Can you work these out from the drawing? Everything is in mm from the part's minimum corner. A direction names the side the tool comes from. Round coordinates to 2 decimals unless told otherwise and drop trailing zeros. Loops run counter-clockwise (first coordinate to the right, second up) from the corner with the lowest first, then second, coordinate; pieces in that order, holes last. Notation, with made-up numbers: M -7,-3.5 L 18,-3.5 A33 cw 18,25.5 Z; hole C 86.25,86.25 d8. An arc over 180 degrees is marked long. Use a Markdown table: item, result.
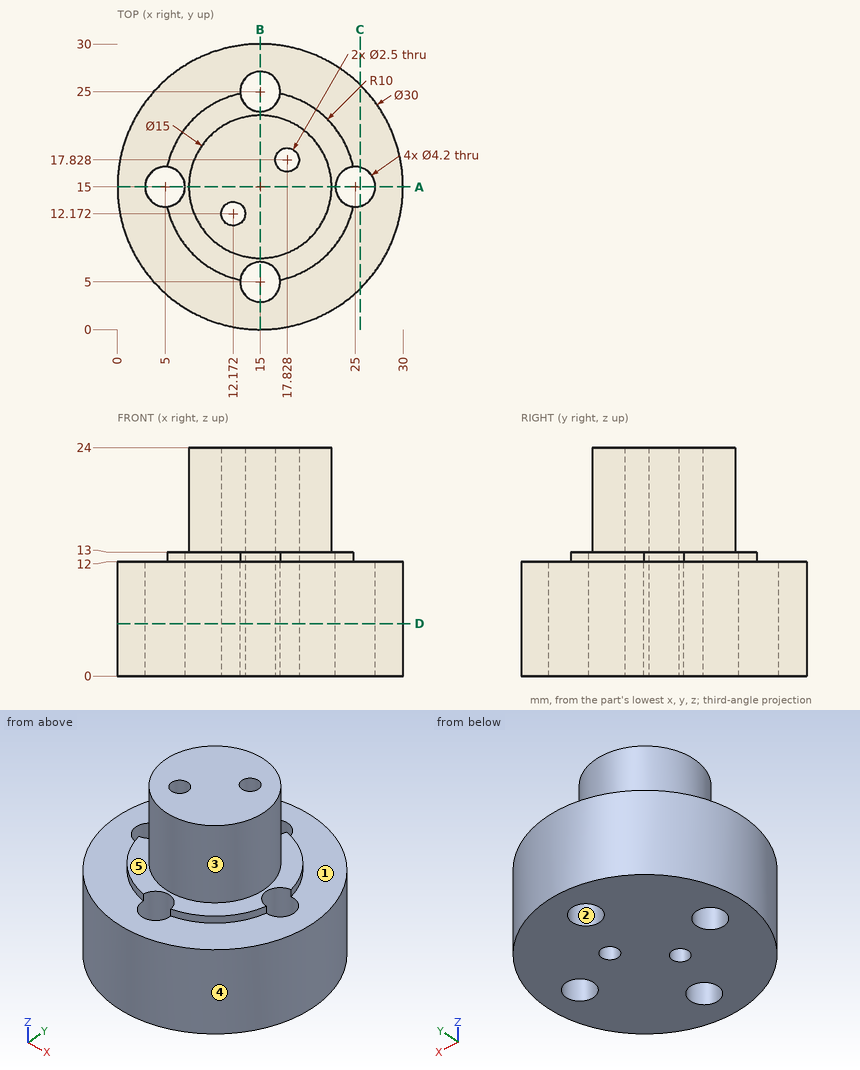
Q1. Imagine slicing it at D-D, the plane z = 5.5. Please give me the cut outline in (x, y).
Return value:
| item | result |
|---|---|
| outline | C 15,15 d30; hole C 5,15 d4.2; hole C 12.17,12.17 d2.5; hole C 15,5 d4.2; hole C 15,25 d4.2; hole C 17.83,17.83 d2.5; hole C 25,15 d4.2 |
Q2. For the marked faces 4 and 5, which set-ups out of +Z, -Z, +X, -X, +Y, -Y let a thin tool reach every point of the face, with its end or its side?
Return value:
| item | result |
|---|---|
| face 4 | +Z, -Z |
| face 5 | +Z |
Q3. Will these pins go through, and if not, where does the flat tip stop? P1, Ø4, axis at y = 7.5, z = 18.5, coming from the +X side; P2, Ø5, axis at y = 21, z = 17.5, coming from the -X side; P3, Ø1.5, axis at y = 9.5, z = 8.5, coming from the +X side; P4, Ø2.5, axis at x = 5, y = 15, coming from the -Z side.
Return value:
| item | result |
|---|---|
| P1 | stops at x = 20.1 |
| P2 | stops at x = 8.37 |
| P3 | stops at x = 29.23 |
| P4 | passes through |
Q4. Imagine slicing it at A-A, the plane y = 15. Please give me the cut outline in (x, z), then the cut area to 3 significant figures.
Return value:
| item | result |
|---|---|
| outline | M 0,0 L 2.9,0 L 2.9,12 L 0,12 Z; M 7.1,0 L 22.9,0 L 22.9,13 L 22.5,13 L 22.5,24 L 7.5,24 L 7.5,13 L 7.1,13 Z; M 27.1,0 L 30,0 L 30,12 L 27.1,12 Z |
| area | 440 mm^2 |
Q5. We'd pull the mould along Y, two halves only. Please class the marked faces 1, 2 and 3: pulls with the +Y half, pulls with the -Y half, needs draft (parallel to the pull), parting line crosses it, or undercut.
Return value:
| item | result |
|---|---|
| face 1 | needs draft |
| face 2 | undercut |
| face 3 | parting line crosses it |
Q6. I need wall thicknesses on line 1 (Y direction, x = 13.5, z = 10.75) (1 decimal); line 2 (Y direction, x = 14.75, z = 22.5) (1 decimal); line 3 (X direction, y = 14, z = 4.25) (1 decimal). Which ranges of each line are inside material? Lowest first, please. Write a range as from..to.
Return value:
| item | result |
|---|---|
| line 1 | y = 0.1..3.5, 6.5..23.5, 26.5..29.9 |
| line 2 | y = 7.5..22.5 |
| line 3 | x = 0..3.2, 6.8..23.2, 26.8..30 |
Q7. Imagine slicing it at C-C, the plane x = 25.5. Please give me the cut outline in (y, z), then the cut area to 3 significant figures.
Return value:
| item | result |
|---|---|
| outline | M 4.29,0 L 12.96,0 L 12.96,12 L 4.29,12 Z; M 17.04,0 L 25.71,0 L 25.71,12 L 17.04,12 Z |
| area | 208 mm^2 |
